```python
from build123d import *

# Parameters (mm, degrees)
SKICA1_W                      = 8.8
SKICA1_H                      = 5.5
SKICA1_W_2                    = 1.9
SKICA1_H_2                    = 4.3
SKICA1_W_3                    = 3.8
SKICA1_H_3                    = 0.25
P_IDAT_VYSUNUT_M1_DEPTH       = 1.6
ZAOBLIT1_R                    = 1
SKICA1_3_W                    = 8.8
SKICA1_3_H                    = 5.5
SKICA1_3_H_2                  = 1.5
P_IDAT_VYSUNUT_M2_DEPTH       = 3
SKICA1_4_W                    = 3.8
SKICA1_4_H                    = 4.8
P_IDAT_VYSUNUT_M3_DEPTH       = 1.7
SKICA1_5_W                    = 7.6
SKICA1_5_H                    = 4.3
P_IDAT_VYSUNUT_M4_DEPTH       = 0.9
ZKOSEN_1_SIZE                 = 0.9
SKICA2_W                      = 4.5
SKICA2_H                      = 3.1
SKICA2_W_2                    = 1.6
SKICA2_H_2                    = 2.9
P_IDAT_VYSUNUT_M5_DEPTH       = 1.2
SKICA2_3_W                    = 7.2
SKICA2_3_H                    = 2.4
SKICA2_3_W_2                  = 3.4
SKICA2_3_H_2                  = 2.3
P_IDAT_VYSUNUT_M6_DEPTH       = 0.8
ZKOSEN_2_SIZE                 = 0.8
SKICA3_W                      = 8
SKICA3_H                      = 2.2
ODEBRAT_VYSUNUT_M1_DEPTH      = 3.6
ZAOBLIT2_R                    = 1
ZKOSEN_3_SIZE                 = 0.8
ZAOBLIT3_R                    = 0.5
SKICA4_W                      = 1.2
SKICA4_H                      = 2.4
P_IDAT_VYSUNUT_M7_DEPTH       = 0.8
SKICA5_W                      = 3
SKICA5_H                      = 1.2
P_IDAT_VYSUNUT_M8_DEPTH       = 0.7
SKICA5_3_W                    = 3
SKICA5_3_H                    = 1.2
P_IDAT_VYSUNUT_M9_DEPTH       = 1.2
SKICA6_W                      = 1.2
SKICA6_H                      = 3.1
P_IDAT_VYSUNUT_M10_DEPTH      = 0.8
SKICA6_3_W                    = 1.2
SKICA6_3_H                    = 4
P_IDAT_VYSUNUT_M11_DEPTH      = 0.9
ZKOSEN_4_SIZE                 = 0.8
P_IDAT_VYSUNUT_M12_DEPTH      = 0.1
P_IDAT_VYSUNUT_M12_DEPTH_BACK = 1.2
SKICA7_W                      = 2.54
SKICA7_H                      = 2.54
SKICA7_R                      = 0.65
SKICA7_2_R                    = 0.65
ODEBRAT_VYSUNUT_M2_DEPTH      = 20.498012719


with BuildPart() as part:
    # Skica1 → Přidat vysunutím1 (new body)
    # profile 1 of 7: a face of its own
    with BuildSketch(Plane.XY):
        Polygon((-9.25, 15.4), (-9.25, -15.4), (-4.4, -15.4), (-4.4, -9.9), (4.4, -9.9), (4.4, -15.4), (9.25, -15.4), (9.25, 15.4), (6.35, 15.4), (6.35, 13.85), (-6.35, 13.85), (-6.35, 15.4), align=None)
        Polygon((-1.9, -0.55), (-1.9, -0.3), (1.9, -0.3), (1.9, -0.55), (3.8, -0.55), (3.8, -4.85), (1.9, -4.85), (1.9, -5.1), (-1.9, -5.1), (-1.9, -4.85), (-3.8, -4.85), (-3.8, -0.55), align=None, mode=Mode.SUBTRACT)
    # profile 2 of 7: a face of its own
    with BuildSketch(Plane.XY):
        with Locations((0, -12.65)):
            Rectangle(SKICA1_W, SKICA1_H)
    # profile 3 of 7: a face of its own
    with BuildSketch(Plane.XY):
        with Locations((2.85, -2.7)):
            Rectangle(SKICA1_W_2, SKICA1_H_2)
    # profile 4 of 7: a face of its own
    with BuildSketch(Plane.XY):
        with Locations((-2.85, -2.7)):
            Rectangle(SKICA1_W_2, SKICA1_H_2)
    # profile 5 of 7: a face of its own
    with BuildSketch(Plane.XY):
        with Locations((0, -2.7)):
            Rectangle(SKICA1_W_3, SKICA1_H_2)
    # profile 6 of 7: a face of its own
    with BuildSketch(Plane.XY):
        with Locations((0, -4.975)):
            Rectangle(SKICA1_W_3, SKICA1_H_3)
    # profile 7 of 7: a face of its own
    with BuildSketch(Plane.XY):
        with Locations((0, -0.425)):
            Rectangle(SKICA1_W_3, SKICA1_H_3)
    extrude(amount=-P_IDAT_VYSUNUT_M1_DEPTH)

    # Zaoblit1
    zaoblit1_edges = [part.edges().sort_by_distance(p)[0] for p in [
        (-6.35, 13.85, -0.8),
        (6.35, 13.85, -0.8),
    ]]
    fillet(zaoblit1_edges, radius=ZAOBLIT1_R)

    # Skica1<3> → Přidat vysunutím2 (add)
    with BuildSketch(Plane.XY):
        with Locations((0, -12.65)):
            Rectangle(SKICA1_3_W, SKICA1_3_H)
        with Locations((0, -16.15)):
            Rectangle(SKICA1_3_W, SKICA1_3_H_2)
    extrude(amount=P_IDAT_VYSUNUT_M2_DEPTH)

    # Skica1<4> → Přidat vysunutím3 (add)
    with BuildSketch(Plane.XY):
        with Locations((0, -2.7)):
            Rectangle(SKICA1_4_W, SKICA1_4_H)
    extrude(amount=P_IDAT_VYSUNUT_M3_DEPTH)

    # Skica1<5> → Přidat vysunutím4 (add)
    with BuildSketch(Plane.XY):
        with Locations((0, -2.7)):
            Rectangle(SKICA1_5_W, SKICA1_5_H)
    extrude(amount=P_IDAT_VYSUNUT_M4_DEPTH)

    # Zkosení1
    zkosen_1_edges = [part.edges().sort_by_distance(p)[0] for p in [
        (-3.8, -2.7, 0.9),
        (3.8, -2.7, 0.9),
    ]]
    chamfer(zkosen_1_edges, length=ZKOSEN_1_SIZE - 0.0001)  # a hair under: the kernel refuses the full size

    # Skica2 → Přidat vysunutím5 (add)
    with BuildSketch(Plane.XY):
        with Locations((2.8, 8.35)):
            Rectangle(SKICA2_W, SKICA2_H)
        with Locations((-4.35, 8.45)):
            Rectangle(SKICA2_W_2, SKICA2_H_2)
    extrude(amount=P_IDAT_VYSUNUT_M5_DEPTH)

    # Skica2<3> → Přidat vysunutím6 (add)
    with BuildSketch(Plane.XY):
        with Locations((2.8, 8.35)):
            Rectangle(SKICA2_3_W, SKICA2_3_H)
        with Locations((-4.35, 8.45)):
            Rectangle(SKICA2_3_W_2, SKICA2_3_H_2)
    extrude(amount=P_IDAT_VYSUNUT_M6_DEPTH)

    # Zkosení2
    zkosen_2_edges = [part.edges().sort_by_distance(p)[0] for p in [
        (6.4, 8.35, 0.8),
        (-0.8, 8.35, 0.8),
        (-2.65, 8.45, 0.8),
        (-6.05, 8.45, 0.8),
    ]]
    chamfer(zkosen_2_edges, length=ZKOSEN_2_SIZE - 0.0001)  # a hair under: the kernel refuses the full size

    # Skica3 → Odebrat vysunutím1 (cut)
    with BuildSketch(Plane.XZ.offset(16.9)):
        with Locations((0, 1.5)):
            Rectangle(SKICA3_W, SKICA3_H)
    extrude(amount=-ODEBRAT_VYSUNUT_M1_DEPTH, mode=Mode.SUBTRACT)

    # Zaoblit2
    zaoblit2_edges = [part.edges().sort_by_distance(p)[0] for p in [
        (4, -15.1, 0.4),
        (-4, -15.1, 0.4),
    ]]
    fillet(zaoblit2_edges, radius=ZAOBLIT2_R)

    # Zkosení3
    zkosen_3_edges = [part.edges().sort_by_distance(p)[0] for p in [
        (4.4, -16.15, 0),
        (-4.4, -16.15, 0),
    ]]
    chamfer(zkosen_3_edges, length=ZKOSEN_3_SIZE)

    # Zaoblit3
    zaoblit3_edges = [part.edges().sort_by_distance(p)[0] for p in [
        (4.4, -13.4, 3),
        (-4.4, -13.4, 3),
    ]]
    fillet(zaoblit3_edges, radius=ZAOBLIT3_R)

    # Skica4 → Přidat vysunutím7 (add)
    with BuildSketch(Plane.XY):
        with Locations((6.05, -3.4)):
            Rectangle(SKICA4_W, SKICA4_H)
        with Locations((6.05, -8.4)):
            Rectangle(SKICA4_W, SKICA4_H)
    extrude(amount=P_IDAT_VYSUNUT_M7_DEPTH)

    # Skica5 → Přidat vysunutím8 (add)
    with BuildSketch(Plane.XY):
        with Locations((-6.15, 4.7)):
            Rectangle(SKICA5_W, SKICA5_H)
        with Locations((4.85, 4.7)):
            Rectangle(SKICA5_W, SKICA5_H)
    extrude(amount=P_IDAT_VYSUNUT_M8_DEPTH)

    # Skica5<3> → Přidat vysunutím9 (add)
    with BuildSketch(Plane.XY):
        with Locations((-2.65, 4.7)):
            Rectangle(SKICA5_3_W, SKICA5_3_H)
        with Locations((-2.65, 2.4)):
            Rectangle(SKICA5_3_W, SKICA5_3_H)
    extrude(amount=P_IDAT_VYSUNUT_M9_DEPTH)

    # Skica6 → Přidat vysunutím10 (add)
    with BuildSketch(Plane.XY):
        with Locations((-6.15, -3.65)):
            Rectangle(SKICA6_W, SKICA6_H)
        with Locations((-6.15, -8.25)):
            Rectangle(SKICA6_W, SKICA6_H)
    extrude(amount=P_IDAT_VYSUNUT_M10_DEPTH)

    # Skica6<3> → Přidat vysunutím11 (add)
    with BuildSketch(Plane.XY):
        with Locations((-7.65, -8.3)):
            Rectangle(SKICA6_3_W, SKICA6_3_H)
        with Locations((-7.65, -3.7)):
            Rectangle(SKICA6_3_W, SKICA6_3_H)
    extrude(amount=P_IDAT_VYSUNUT_M11_DEPTH)

    # Zkosení4
    zkosen_4_edges = [part.edges().sort_by_distance(p)[0] for p in [
        (-7.65, -6.3, 0.9),
        (-7.65, -10.3, 0.9),
        (-7.65, -1.7, 0.9),
        (-7.65, -5.7, 0.9),
    ]]
    chamfer(zkosen_4_edges, length=ZKOSEN_4_SIZE)

    # Skica7 → Přidat vysunutím12 (add, two sides: drawn at the far end of the back side and taken through both)
    # profile 1 of 6: a face of its own
    with BuildSketch(Plane.XY.offset(-P_IDAT_VYSUNUT_M12_DEPTH_BACK)):
        with Locations((-7.48, 12.03)):
            Rectangle(SKICA7_W, SKICA7_H)
        with Locations((-7.48, 12.03)):
            Circle(SKICA7_R, mode=Mode.SUBTRACT)
    # profile 2 of 6: a face of its own
    with BuildSketch(Plane.XY.offset(-P_IDAT_VYSUNUT_M12_DEPTH_BACK)):
        with Locations((-4.52, 12.03)):
            Rectangle(SKICA7_W, SKICA7_H)
        with Locations((-4.52, 12.03)):
            Circle(SKICA7_R, mode=Mode.SUBTRACT)
    # profile 3 of 6: a face of its own
    with BuildSketch(Plane.XY.offset(-P_IDAT_VYSUNUT_M12_DEPTH_BACK)):
        with Locations((-7.48, -13.63)):
            Rectangle(SKICA7_W, SKICA7_H)
        with Locations((-7.48, -13.63)):
            Circle(SKICA7_R, mode=Mode.SUBTRACT)
    # profile 4 of 6: a face of its own
    with BuildSketch(Plane.XY.offset(-P_IDAT_VYSUNUT_M12_DEPTH_BACK)):
        with Locations((7.48, -13.63)):
            Rectangle(SKICA7_W, SKICA7_H)
        with Locations((7.48, -13.63)):
            Circle(SKICA7_R, mode=Mode.SUBTRACT)
    # profile 5 of 6: a face of its own
    with BuildSketch(Plane.XY.offset(-P_IDAT_VYSUNUT_M12_DEPTH_BACK)):
        with Locations((4.52, 12.03)):
            Rectangle(SKICA7_W, SKICA7_H)
        with Locations((4.52, 12.03)):
            Circle(SKICA7_R, mode=Mode.SUBTRACT)
    # profile 6 of 6: a face of its own
    with BuildSketch(Plane.XY.offset(-P_IDAT_VYSUNUT_M12_DEPTH_BACK)):
        with Locations((7.48, 12.03)):
            Rectangle(SKICA7_W, SKICA7_H)
        with Locations((7.48, 12.03)):
            Circle(SKICA7_R, mode=Mode.SUBTRACT)
    extrude(amount=P_IDAT_VYSUNUT_M12_DEPTH + P_IDAT_VYSUNUT_M12_DEPTH_BACK)

    # Skica7<2> → Odebrat vysunutím2 (cut, through all)
    with BuildSketch(Plane.XY):
        with Locations((-7.48, -13.63)):
            Circle(SKICA7_2_R)
        with Locations((7.48, -13.63)):
            Circle(SKICA7_2_R)
        with Locations((-7.48, 12.03)):
            Circle(SKICA7_2_R)
        with Locations((-4.52, 12.03)):
            Circle(SKICA7_2_R)
        with Locations((4.52, 12.03)):
            Circle(SKICA7_2_R)
        with Locations((7.48, 12.03)):
            Circle(SKICA7_2_R)
    extrude(amount=-ODEBRAT_VYSUNUT_M2_DEPTH, mode=Mode.SUBTRACT)


solid = part.part
```
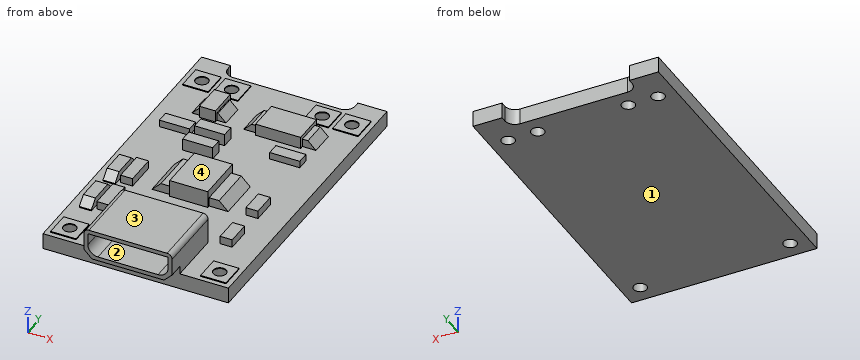
Could you check a few things on this model? Use its own coordinates, in mm. Face numbers are marked on the shaded views. A direction names the side the tool comes from. Coordinates: 2 decimals unless noted, no trailing zeros. Write each loop counter-clockwise with the first axis right and the second up, starting at its lowest first coordinate (ties: lowest second). Pieces come first, ordered by that corner, then holes. Notation, with made-up numbers: M -3,8.5 L 24,8.5 A27 ccw 24,33.5 Z; hole C 44.25,47 d10. An arc over 180 degrees is marked long. Answer as CSV lines item,"result". Start each with the question number.
1) We'd pull the mould along X, two halves only. Please class the marked faces 1 and 2: +X half, -X half, draft (parallel to the pull), parting line (faces both ways), or undercut.
2) I want a section at B-B, the plane x = 7.48. Please give me the cut outline in (y, z).
3) I want a section at C-C, the plane y = 4.5. Please give me the cut outline in (x, z), and give its area (3 significant figures).
4) Please list where these lines run through material, in increasing order: line 1 (X direction, y = 12.03, z = -1.2); line 2 (Y direction, x = 7.48, z = 0.05); line 3 (Y direction, x = -7.48, z = -1). Write a range as from..to.
5) For the marked faces 3 and 4, which set-ups out of +Z, -Z, +X, -X, +Y, -Y let a thin tool reach every point of the face, with its end or its side?
6) I want a section at A-A, the plane y = -13.63. Give the number of separate pieces and of enclosed holes in the cut face, and give its area (3 significant figures).
7) I want a section at D-D, the plane x = 2.25. Please give me the cut outline in (y, z), and give its area (3 significant figures).
8) For P1, Ø5, axis at x = 0, y = -7, coming from the +Z side; P2, Ø3.5, axis at x = 4, y = 8, coming from the +Z side; P3, Ø2, axis at x = 3.5, z = 0.5, coming from the +Y side, each with a flat end and sliding along its axis, tell me the tip position at first contact or that it passes through.
Data:
1,face 1,"draft"
1,face 2,"undercut"
2,outline,"M -15.4,-1.6 L -14.28,-1.6 L -14.28,0.1 L -14.9,0.1 L -14.9,0 L -15.4,0 Z; M -12.98,-1.6 L 11.38,-1.6 L 11.38,0.1 L 10.76,0.1 L 10.76,0 L -12.36,0 L -12.36,0.1 L -12.98,0.1 Z; M 12.68,-1.6 L 15.4,-1.6 L 15.4,0 L 13.3,0 L 13.3,0.1 L 12.68,0.1 Z"
3,outline,"M -9.25,-1.6 L 9.25,-1.6 L 9.25,0 L 6.35,0 L 6.35,0.7 L 3.35,0.7 L 3.35,0 L -1.15,0 L -1.15,1.2 L -4.15,1.2 L -4.15,0 L -4.65,0 L -4.65,0.7 L -7.65,0.7 L -7.65,0 L -9.25,0 Z"
3,area,"37.4 mm^2"
4,line 1,"x = -9.25..-8.13, -6.83..-5.17, -3.87..3.87, 5.17..6.83, 8.13..9.25"
4,line 2,"y = -14.9..-14.28, -12.98..-12.36, 10.76..11.38, 12.68..13.3"
4,line 3,"y = -15.4..-14.28, -12.98..11.38, 12.68..15.4"
5,face 3,"+Z, +X, -X, +Y, -Y"
5,face 4,"+Z, +X, -X, +Y"
6,separate pieces,"3"
6,enclosed holes,"1"
6,area,"34.8 mm^2"
7,outline,"M -16.9,0 L -15.4,0 L -15.4,-1.6 L 13.85,-1.6 L 13.85,0 L 9.9,0 L 9.9,1.2 L 6.8,1.2 L 6.8,0 L -0.55,0 L -0.55,0.9 L -4.85,0.9 L -4.85,0 L -9.9,0 L -9.9,3 L -16.9,3 L -16.9,2.6 L -13.3,2.6 L -13.3,0.4 L -16.9,0.4 Z"
7,area,"67.5 mm^2"
8,P1,"stops at z = 1.7"
8,P2,"stops at z = 1.2"
8,P3,"stops at y = 13.85"
